Verification items for the finished model (mm, model axes). A direction names the side the tool comes from. Coordinates: 2 decimals unless noted, no trailing zeros. Write each loop counter-clockwise with the first axis right and the second up, starting at its lowest first coordinate (ties: lowest second). Pieces come first, ordered by that corner, then holes. Notation, with made-up numbers: (-34, -34.5) -> (0, -34.5) arc R20 cw to (0, -28.5) -> close; hole circle Ø5 at (42, -15). An arc over 180 degrees is marked (long way). Use CSV: the item, a comma, the result in double quotes.
```python
from build123d import *

# Parameters (mm, degrees)
SKETCH1_W               = 270
SKETCH1_H               = 30
BOSS_EXTRUDE1_DEPTH     = 15
CUT_EXTRUDE1_REACH      = 274.075
SKETCH2_W               = 35
SKETCH2_H               = 15
CUT_EXTRUDE2_DEPTH      = 274.313007374
CUT_EXTRUDE2_DEPTH_BACK = 274.313007374
SKETCH3_R               = 5
FILLET3_R               = 15


with BuildPart() as part:
    # Sketch1 → Boss-Extrude1 (new, symmetric)
    with BuildSketch(Plane.XY):
        with Locations((135, 15)):
            Rectangle(SKETCH1_W, SKETCH1_H)
    extrude(amount=BOSS_EXTRUDE1_DEPTH, both=True)

    # Sketch2 → Cut-Extrude1 (cut, up to next)
    with BuildSketch(Plane(origin=(0, 30, 0), x_dir=(1, 0, 0), z_dir=(0, 1, 0)), mode=Mode.PRIVATE) as cut_extrude1_sk1:
        with Locations((252.5, 0)):
            Rectangle(SKETCH2_W, SKETCH2_H)
    cut_extrude1_tool1 = extrude(cut_extrude1_sk1.sketch, amount=-CUT_EXTRUDE1_REACH, mode=Mode.PRIVATE) & part.part
    add(cut_extrude1_tool1.solids().sort_by_distance((252.5, 30, 0))[0], mode=Mode.SUBTRACT)

    # Sketch3 → Cut-Extrude2 (cut, two sides: drawn at the far end of the back side and taken through both)
    with BuildSketch(Plane.XY.offset(15).offset(-CUT_EXTRUDE2_DEPTH_BACK)):
        with Locations((15, 15)):
            Circle(SKETCH3_R)
        with Locations((255, 15)):
            Circle(SKETCH3_R)
        with Locations((125, 15)):
            Circle(SKETCH3_R)
    extrude(amount=CUT_EXTRUDE2_DEPTH + CUT_EXTRUDE2_DEPTH_BACK, mode=Mode.SUBTRACT)

    # Fillet3
    fillet3_edges = [part.edges().sort_by_distance(p)[0] for p in [
        (270, 0, -11.25),
        (270, 30, -11.25),
        (270, 0, 11.25),
        (270, 30, 11.25),
        (0, 0, 0),
        (0, 30, 0),
    ]]
    fillet(fillet3_edges, radius=FILLET3_R - 0.0001)  # a hair under: the kernel refuses the full size


solid = part.part
```
1) Cross-section at D-D (y = 3.5). Record the boundary of the cut face in (x, z).
Return value:
outline,"(5.37, -15) -> (264.63, -15) -> (264.63, -7.5) -> (235, -7.5) -> (235, 7.5) -> (264.63, 7.5) -> (264.63, 15) -> (5.37, 15) -> close"
2) Cross-section at B-B (z = -4.5). Give the number of separate pieces and of enclosed holes in the cut face, plus the area to 3 significant figures.
Return value:
separate pieces,"1"
enclosed holes,"2"
area,"6,800 mm2"
3) Cross-section at A-A (x = 125). Record the boundary of the cut face in (y, z).
Return value:
outline,"(0, -15) -> (10, -15) -> (10, 15) -> (0, 15) -> close; (20, -15) -> (30, -15) -> (30, 15) -> (20, 15) -> close"
4) Gauge pin test, flat ends, axial feed: pin 1 (7.5 mm diameter, centred on y = 16.5, z = 1.5, fed in from +X); pin 2 (4 mm diameter, centred on y = 6, z = -7, fed in from +X); pin 3 (5 mm diameter, centred on y = 7, z = -10, fed in from -X); pin 4 (6 mm diameter, centred on x = 125, y = 15, fed in from +Z). Record the tip position at first contact, or that the pin passes through.
Return value:
pin 1,"x = 235"
pin 2,"x = 268.23"
pin 3,"x = 1.04"
pin 4,"through"
5) Mould release check, pull along Z, two halves, no side actions. Record for faces 1 (the flat face through (133, 15, 15)), 2 (the flat face through (133, 15, -15)), 3 (the cylindrical face through (259.619, 13.085, 11.197)), 4 (the flat face through (248, 15, 7.5)): released by +Z, released by -Z, zero draft, split by the parting line, or undercut.
Return value:
face 1,"released by +Z"
face 2,"released by -Z"
face 3,"zero draft"
face 4,"undercut"
6) Set-up check for faces 5 (the cylindrical face through (265.49, 4.28, -11.2)), 6 (the flat face through (235, 15, 0)): record each of +Z, -Z, +X, -X, +Y, -Y from which the full face is reachable in a straight line by a thin tool's end or side.
Return value:
face 5,"+Z, -Z, +X, -Y"
face 6,"+X, +Y, -Y"
7) Cross-section at C-C (y = 27.5). Record the boundary of the cut face in (x, z).
Return value:
outline,"(6.71, -15) -> (263.29, -15) -> (263.29, -7.5) -> (235, -7.5) -> (235, 7.5) -> (263.29, 7.5) -> (263.29, 15) -> (6.71, 15) -> close"
8) Scan lines: L1, parallel to X at y = 15, z = 11.25; L2, parallel to X at y = 15, z = 4; L3, parallel to Y at x = 125, z = -0.75. Record each from-to range of solid material in increasing order.
Return value:
L1,"0 to 10, 20 to 120, 130 to 250, 260 to 270"
L2,"0 to 10, 20 to 120, 130 to 235"
L3,"0 to 10, 20 to 30"
